```python
from build123d import *

# Parameters (mm, degrees)
F0_W     = 47.2308259338
F0_H     = 127.08
F0_W_2   = 2.84589082
F0_H_2   = 8
F0_W_3   = 73.3691740662
F0_W_4   = 2.6096887887
F1_DEPTH = 7.9756
F3_W     = 30.1258238032
F3_H     = 46.3937623426
F4_DEPTH = 6.35
F6_W     = 9.6924505796
F6_H     = 2.8718380383
F7_DEPTH = 25.4
F8_DEPTH = 12.7


with BuildPart() as f1:
    # F0 (on Top) → F1 (new body)
    with BuildSketch(Plane.XY):
        with Locations((-23.6154129669, -4.7186717279)):
            Rectangle(F0_W, F0_H)
        with Locations((-38.4195260704, -4.7210717279)):
            Rectangle(F0_W_2, F0_H_2, mode=Mode.SUBTRACT)
        with Locations((36.6845870331, -4.7186717279)):
            Rectangle(F0_W_3, F0_H)
        with Locations((60.218263734, -4.7210717279)):
            Rectangle(F0_W_4, F0_H_2, mode=Mode.SUBTRACT)
    extrude(amount=F1_DEPTH)

    # F3 (on offset) → F4 (join)
    with BuildSketch(Plane.XZ.offset(68.2586717279)):
        with Locations((10.9603698365, -14.6902077831)):
            Rectangle(F3_W, F3_H)
    extrude(amount=F4_DEPTH)

    # F6 (on offset) → F7 (join)
    with BuildSketch(Plane(origin=(0, 0, 0), x_dir=(1, 0, 0), z_dir=(0, 0, -1))):
        with Locations((11.2944499124, 61.5227527088)):
            Rectangle(F6_W, F6_H)
        Polygon((6.4482246226, 60.0868336896), (6.4482246226, 62.9586717279), (-3.9315340109, 62.9586717279), (-3.9315340109, 55.2566833794), (25.8039161563, 55.2566833794), (25.8039161563, 62.9586717279), (16.1406752022, 62.9586717279), (16.1406752022, 60.0868336896), align=None)
    extrude(amount=F7_DEPTH)

    # F8 (add): a face of the model
    f8_faces = [f1.faces().sort_by_distance(p)[0] for p in [
        (10.9361910727, -59.1076775537, -25.4),
    ]]
    extrude(f8_faces, amount=F8_DEPTH)


solid = f1.part
```
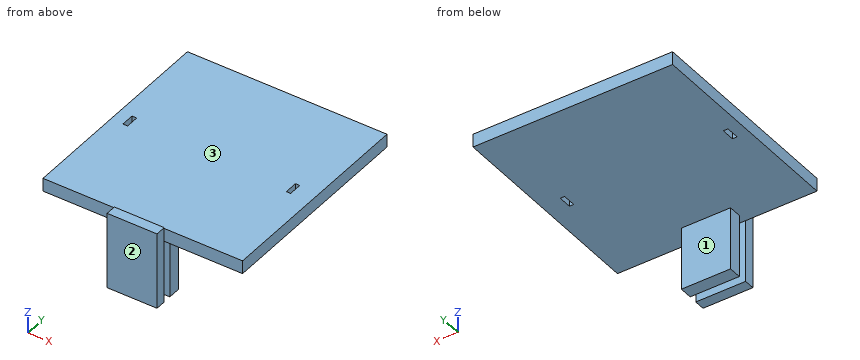
Here's how the part is built. I have some questions about the finished solid (model axes, mm). Face numbers are marked on the shaded views. A direction names the side the tool comes from. Coordinates: 2 decimals unless noted, no trailing zeros. Write each loop counter-clockwise with the first axis right and the second up, starting at its lowest first coordinate (ties: lowest second). Pieces come first, ordered by that corner, then holes. Notation, with made-up numbers: (-26, 54) -> (7, 54) arc R30 ccw to (7, 92) -> close; hole circle Ø10 at (52.25, 53.25). An arc over 180 degrees is marked (long way). Use a Markdown table: item, result. Add a question column.
(1) If we section it at C-C, the plane y = 45.5: Write out the boundary of the cut face in (x, z), and give its area (3 significant figures).
(2) I'm going to push flat-ended pins straight in: P1, Ø6, axis at y = -58, z = -11.5, coming from the -X side; P2, Ø2, axis at x = 23.5, z = -17, coming from the +Y side; P3, Ø8.5, axis at y = -58.5, z = -20.5, coming from the +X side. Where does each tip first touch, or does it pass through?
(3) If we section it at A-A, the plane z = -10.5: Write out the boundary of the cut face in (x, y), and give its area (3 significant figures).
(4) If we section it at B-B, the plane x = 10: Write out the boundary of the cut face in (y, z), and give its area (3 significant figures).
(5) If we section it at D-D, the plane x = 38: Write out the boundary of the cut face in (y, z).
(6) For the marked faces 1, 2 and 3, which set-ups out of +Z, -Z, +X, -X, +Y, -Y let a thin tool reach every point of the face, with its end or its side?
(7) Please list where these lines run through material, in increasing order: line 1 (Y direction, x = -1.5, z = -1.5); line 2 (Z direction, x = -34, y = 12.5); line 3 (Y direction, x = 38, z = 4.5).
Outcome:
| question | item | result |
|---|---|---|
| 1 | outline | (-47.23, 0) -> (73.37, 0) -> (73.37, 7.98) -> (-47.23, 7.98) -> close |
| 1 | area | 962 mm^2 |
| 2 | P1 | stops at x = -3.93 |
| 2 | P2 | stops at y = -55.26 |
| 2 | P3 | stops at x = 25.8 |
| 3 | outline | (-4.1, -74.61) -> (26.02, -74.61) -> (26.02, -68.26) -> (-4.1, -68.26) -> close; (-3.93, -62.96) -> (25.8, -62.96) -> (25.8, -55.26) -> (-3.93, -55.26) -> close |
| 3 | area | 420 mm^2 |
| 4 | outline | (-74.61, -37.89) -> (-68.26, -37.89) -> (-68.26, 0) -> (-62.96, 0) -> (-62.96, -38.1) -> (-55.26, -38.1) -> (-55.26, 0) -> (58.82, 0) -> (58.82, 7.98) -> (-68.26, 7.98) -> (-68.26, 8.51) -> (-74.61, 8.51) -> close |
| 4 | area | 1,600 mm^2 |
| 5 | outline | (-68.26, 0) -> (58.82, 0) -> (58.82, 7.98) -> (-68.26, 7.98) -> close |
| 6 | face 1 | -Z, +X, -X, +Y |
| 6 | face 2 | +Z, -Z, +X, -X, -Y |
| 6 | face 3 | +Z, +X, -X, +Y |
| 7 | line 1 | y = -74.61 to -68.26, -62.96 to -55.26 |
| 7 | line 2 | z = 0 to 7.98 |
| 7 | line 3 | y = -68.26 to 58.82 |
